Check sheet for the modelled part. Datum: model origin and axes. Units: mm. Face numbers are marked on the shaded views. A direction names the side the tool comes from. Round coordinates to 2 decimals unless told otherwise and drop trailing zeros. Write each loop counter-clockwise with the first axis right and the second up, starting at its lowest first coordinate (ties: lowest second). Pieces come first, ordered by that corner, then holes. Notation, with made-up numbers: M 66,24 L 108,24 A13 ccw 108,37 Z; hole C 3,1.25 d2. An arc over 180 degrees is marked long. Put each result on its own line as item: value.
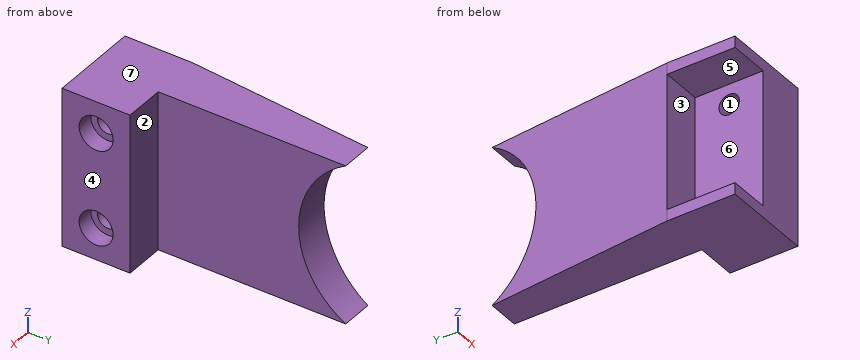
```python
from build123d import *

# Parameters (mm, degrees)
GRIPPER_ATTACHMENT_BASE_SKETCH_W = 11.1125
GRIPPER_ATTACHMENT_BASE_SKETCH_H = 15
GRIPPER_ATTACHMENT_BASE_DEPTH    = 35.0588586
THROUGH_HOLES_SKETCH_R           = 2.25
SCREW_THROUGH_HOLES_DEPTH        = 38.534800154
SOCKET_RECESSES_SKETCH_R         = 3.75
SOCKET_RECESSES_DEPTH            = 3.75
FINGER_CAVITY_SKETCH_W           = 2.5294293
FINGER_CAVITY_SKETCH_H           = 15
FINGER_CAVITY_DEPTH              = 9
THICKENER_BASE_DEPTH             = 11.1125
THICKNESS_CUTOFF_SKETCH_W        = 61.996732773
THICKNESS_CUTOFF_SKETCH_H        = 64.835459205
THICKNESS_CUTOFF_DEPTH           = 63.508667222


with BuildPart() as part:
    # Gripper Attachment Base Sketch → Gripper Attachment Base (new body)
    with BuildSketch(Plane.XY):
        Rectangle(GRIPPER_ATTACHMENT_BASE_SKETCH_W, GRIPPER_ATTACHMENT_BASE_SKETCH_H)
    extrude(amount=GRIPPER_ATTACHMENT_BASE_DEPTH)

    # Through-Holes Sketch → Screw Through-Holes (cut, through all)
    with BuildSketch(Plane(origin=(5.55625, 0, 0), x_dir=(0, 0, -1), z_dir=(1, 0, 0))):
        with Locations(Location((-28.0294293, 0, 0), (0, 0, 90))):
            Circle(THROUGH_HOLES_SKETCH_R)
        with Locations(Location((-7.0294293, 0, 0), (0, 0, 90))):
            Circle(THROUGH_HOLES_SKETCH_R)
    extrude(amount=-SCREW_THROUGH_HOLES_DEPTH, mode=Mode.SUBTRACT)

    # Socket Recesses Sketch → Socket Recesses (cut)
    with BuildSketch(Plane(origin=(5.55625, 0, 0), x_dir=(0, 0, -1), z_dir=(1, 0, 0))):
        with Locations(Location((-28.0294293, 0, 0), (0, 0, 90))):
            Circle(SOCKET_RECESSES_SKETCH_R)
        with Locations(Location((-7.0294293, 0, 0), (0, 0, 90))):
            Circle(SOCKET_RECESSES_SKETCH_R)
    extrude(amount=-SOCKET_RECESSES_DEPTH, mode=Mode.SUBTRACT)

    # Finger Cavity Sketch → Finger Cavity (add)
    with BuildSketch(Plane.ZY.offset(5.55625)):
        with Locations((1.26471465, 0)):
            Rectangle(FINGER_CAVITY_SKETCH_W, FINGER_CAVITY_SKETCH_H)
        with Locations((33.79414395, 0)):
            Rectangle(FINGER_CAVITY_SKETCH_W, FINGER_CAVITY_SKETCH_H)
    extrude(amount=FINGER_CAVITY_DEPTH)

    # Thickener Base Sketch → Thickener Base (add)
    with BuildSketch(Plane(origin=(-3.44375, 0, 0), x_dir=(0, 0, -1), z_dir=(1, 0, 0))):
        with BuildLine():
            Line((0, 7.5), (-35.0588586, 7.5))
            Line((-35.0588586, 7.5), (-35.0588586, 48.89593))
            ThreePointArc((-35.0588586, 48.89593), (-17.5294293, 38.525006197), (0, 48.89593))
            Line((0, 48.89593), (0, 7.5))
        make_face()
    extrude(amount=-THICKENER_BASE_DEPTH)

    # Thickness Cutoff Sketch → Thickness Cutoff (cut, through all)
    with BuildSketch(Plane(origin=(-15.139601336, 1.462907231, 0), x_dir=(0, 0, -1), z_dir=(0.9953639682653084, -0.09617988708216554, 0))):
        with Locations((-17.347442804, 24.375229456)):
            Rectangle(THICKNESS_CUTOFF_SKETCH_W, THICKNESS_CUTOFF_SKETCH_H)
    extrude(amount=-THICKNESS_CUTOFF_DEPTH, mode=Mode.SUBTRACT)


solid = part.part
```
1. Release check for a two-part mould opening along Z. For the marked faces 4, 5, 6 and 7 record: +Z half, -Z half, draft (parallel to the pull), parting line (faces both ways), or undercut.
Computed values:
face 4: draft
face 5: undercut
face 6: undercut
face 7: +Z half
2. Cross-section at A-A (y = 0). Enter the section's corners in (x, z), then the cut area to 3 significant figures.
Computed values:
outline: M -14.56,0 L 5.56,0 L 5.56,3.28 L 1.81,3.28 L 1.81,4.78 L -5.56,4.78 L -5.56,2.53 L -14.56,2.53 Z; M -14.56,32.53 L -5.56,32.53 L -5.56,30.28 L 1.81,30.28 L 1.81,31.78 L 5.56,31.78 L 5.56,35.06 L -14.56,35.06 Z; M -5.56,9.28 L 1.81,9.28 L 1.81,10.78 L 5.56,10.78 L 5.56,24.28 L 1.81,24.28 L 1.81,25.78 L -5.56,25.78 Z
area: 313 mm2
3. Cross-section at C-C (z = 22.5). Enter the section's corners in (x, y).
Computed values:
outline: M -14.56,7.5 L -5.56,7.5 L -5.56,-7.5 L 5.56,-7.5 L 5.56,7.5 L -3.44,7.5 L -3.44,39.15 L -11.5,39.15 Z
4. Depth check by flat-ended pin: pin 1 Ø6 at (y, z) = (-0.5, 5) entering from +X; pin 2 Ø1 at (y, z) = (36, 13) entering from -X; pin 3 Ø3 at (y, z) = (22.5, 23) entering from -X; pin 4 Ø6 at (y, z) = (14.5, 14) entering from +X. Enter the tip coordinate at first touch or a pass-through.
Computed values:
pin 1: stops at x = 5.56
pin 2: stops at x = -11.85
pin 3: stops at x = -13.25
pin 4: stops at x = -3.44
5. Cross-section at D-D (x = 0.5). Enter the section's corners in (y, z), then the cut area to 3 significant figures.
Computed values:
outline: M -7.5,0 L 7.5,0 L 7.5,35.06 L -7.5,35.06 Z; hole C 0,7.03 d4.5; hole C 0,28.03 d4.5
area: 494 mm2
6. Scan lines: probe 1 along Z at (x, y) = (2.6, 0); probe 2 along Z at (x, y) = (-0.25, 0); probe 3 along X at (y, z) = (2.5, 10). Record each from-to range of solid material in increasing order.
Computed values:
probe 1: z = 0 to 3.28, 10.78 to 24.28, 31.78 to 35.06
probe 2: z = 0 to 4.78, 9.28 to 25.78, 30.28 to 35.06
probe 3: x = -5.56 to 5.56
7. Cross-section at B-B (x = -6.75). Enter the section's corners in (y, z) (3 decimals).
Computed values:
outline: M -7.5,0 L 48.896,0 A20 cw 48.896,35.059 L -7.5,35.059 L -7.5,32.529 L 7.5,32.529 L 7.5,2.529 L -7.5,2.529 Z
8. Access from +Z, -Z, +X, -X, +Y, -Y to the whole of each face (thin tool, end or side, straight path). Record for the marked faces 1, 2 and 3.
Computed values:
face 1: +X, -X
face 2: +Z, -Z, +X, +Y
face 3: -X, -Y
